```python
from build123d import *

# Parameters (mm, degrees)
SKETCH1_W           = 30
SKETCH1_H           = 60
BOSS_EXTRUDE1_DEPTH = 60
CUT_EXTRUDE1_DEPTH  = 60
SKETCH4_W           = 20
SKETCH4_H           = 40
CUT_EXTRUDE2_DEPTH  = 60
CUT_EXTRUDE3_DEPTH  = 60
BOSS_EXTRUDE2_DEPTH = 20
CUT_EXTRUDE9_DEPTH  = 20


with BuildPart() as part:
    # Sketch1 → Boss-Extrude1 (new body)
    with BuildSketch(Plane.XY):
        with BuildLine():
            ThreePointArc((30, 60), (60, 30), (30, 0))
            Line((30, 0), (30, 60))
        make_face()
        with Locations((15, 30)):
            Rectangle(SKETCH1_W, SKETCH1_H)
    extrude(amount=BOSS_EXTRUDE1_DEPTH)

    # Sketch2 → Cut-Extrude1 (cut)
    with BuildSketch(Plane.ZY):
        Polygon((0, 60), (60, 0), (60, 60), align=None)
    extrude(amount=-CUT_EXTRUDE1_DEPTH, mode=Mode.SUBTRACT)

    # Sketch4 → Cut-Extrude2 (cut)
    with BuildSketch(Plane(origin=(0, 0, 0), x_dir=(-1, 0, 0), z_dir=(0, 0, -1))):
        with Locations((-10.0001, 30)):
            Rectangle(SKETCH4_W, SKETCH4_H)
    extrude(amount=-CUT_EXTRUDE2_DEPTH, mode=Mode.SUBTRACT)

    # Sketch5 → Cut-Extrude3 (cut)
    with BuildSketch(Plane(origin=(0, 0, 0), x_dir=(-1, 0, 0), z_dir=(0, 0, -1))):
        with BuildLine():
            Line((-30, 50), (-20.0003, 50))
            Line((-20.0003, 50), (-20.0003, 10.000000002))
            Line((-20.0003, 10.000000002), (-30.0003, 10.000000002))
            ThreePointArc((-30.0003, 10.000000002), (-49.999999999, 30.00015), (-30, 50))
        make_face()
    extrude(amount=-CUT_EXTRUDE3_DEPTH, mode=Mode.SUBTRACT)

    # Sketch6 → Boss-Extrude2 (add)
    with BuildSketch(Plane.ZY.offset(-20.0001)):
        Polygon((0, 50.000000001), (9.999999999, 50.000000001), (50, 10), (0, 10), align=None)
    extrude(amount=BOSS_EXTRUDE2_DEPTH)

    # Sketch7 → Cut-Extrude9 (cut)
    with BuildSketch(Plane.ZY):
        Polygon((49.999999998, 10.000000002), (49.996907355, 10.000000002), (0.748306112, 50), (10, 50), align=None)
    extrude(amount=-CUT_EXTRUDE9_DEPTH, mode=Mode.SUBTRACT)


solid = part.part
```
The listing builds one solid part. Answer for the finished solid, in the listing's coordinates (mm). A direction names the side the tool comes from. Give positions to 0.01 mm unless a question says otherwise; leave off trailing zeros. Order: outer loops, then holes, each group sorted by start corner. A loop starts at its lowest first (then second) coordinate and runs counter-clockwise, first axis right, second up.
1) Find section A-A on x = 40. Write down the section's boundary in (y, z).
Reported:
outline: (1.72, 0) - (12.68, 0) - (12.68, 47.32) - (1.72, 58.28) - close; (47.32, 0) - (58.28, 0) - (58.28, 1.72) - (47.32, 12.68) - close
2) Determine the mould class of faces 4 (the face through (0, 16, 23)), 5 (the face through (53.4, 11.226, 22.913)), 6 (the face through (25, 10, 25)), 7 (the face through (15, 0, 30)) for opening direction X: pulls with the +X half, pulls with the -X half, needs draft (parallel to the pull), parting line crosses it, or undercut.
Reported:
face 4: pulls with the -X half
face 5: pulls with the +X half
face 6: undercut
face 7: needs draft
3) For faces 1 (the face through (9.86, 29.72, 25.72)), 2 (the face through (50.4, 30.4, 29.6)), 3 (the face through (48.64, 22.75, 19.09)), determine the directions among +Z, -Z, +X, -X, +Y, -Y from which every point of the face is accessible in a straight line to the end or side of a thin tool.
Reported:
face 1: +Z, -X
face 2: +Z, +X, -X, +Y
face 3: +Z, -Z
4) Find section D-D on z = 5. Write down the section's boundary in (x, y).
Reported:
outline: (0, 0) - (30, 0) arc R30 ccw to (46.58, 55) - (0, 55) - (0, 50) - (20, 50) - (20, 46.55) - (0, 46.55) - close; hole (20, 10) - (30, 10) arc R20 ccw to (30, 50) - (20, 50) - close
5) Consider line 1 along Y through (x, z) = (23, 25); line 2 along X through (y, z) = (39, 8); line 3 along Y through (x, z) = (33.5, 9). Determine where each line is inside the solid, lowest interval first.
Reported:
line 1: y = 0 to 10
line 2: x = 0 to 20, 47.86 to 58.62
line 3: y = 0.2 to 10.31, 49.69 to 51
6) Given P1, Ø4, axis at x = 13.5, y = 41, coming from the +Z side; P2, Ø6, axis at x = 36, z = 48, coming from the +Y side; P3, Ø12, axis at x = 24, y = 9.5, coming from the +Z side, each flat-ended and moving along its own axis, determine where each tip first touches the part or whether it passes through.
Reported:
P1: stops at z = 14.29
P2: stops at y = 12.14
P3: stops at z = 56.5
